Could you check a few things on this model? Use its own coordinates, in mm. Face numbers are marked on the shaded views. A direction names the side the tool comes from. Coordinates: 2 decimals unless noted, no trailing zeros. Write each loop counter-clockwise with the first axis right and the second up, starting at its lowest first coordinate (ties: lowest second). Pieces come first, ordered by that corner, then holes.
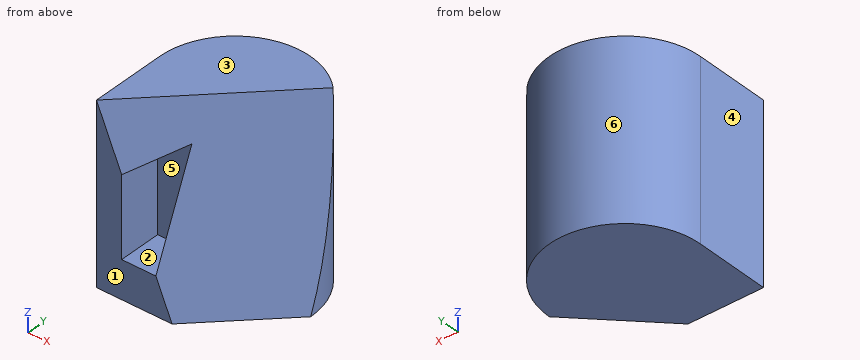
```python
from build123d import *

# Parameters (mm, degrees)
F1_DEPTH = 70
F6_DEPTH = 25


with BuildPart() as f1:
    # F0 (on Top) → F1 (new body)
    with BuildSketch(Plane.XY):
        with BuildLine():
            Line((-30, 0), (-30, -30))
            Line((-30, -30), (0, -30))
            Line((0, -30), (30, 0))
            ThreePointArc((30, 0), (0, 30), (-30, 0))
        make_face()
    extrude(amount=F1_DEPTH)

    # F4: sweep along a path in F3
    with BuildLine(Plane.XY.offset(70)) as f4_path:
        Line((-30, -30), (0, 0))
        Line((0, 0), (21.2132034356, 21.2132034356))
    # F2 (on face) → F4 (sweep, cut)
    with BuildSketch(Plane.XZ.offset(30)):
        Polygon((0, 70), (-30, 70), (0, 0), align=None)
    sweep(path=f4_path.line, mode=Mode.SUBTRACT)

    # F5 (on face) → F6 (cut)
    with BuildSketch(Plane.XZ.offset(30)):
        Polygon((-20, 46.6666666667), (-20, 15), (-6.4285714286, 15), (-6.4285714286, 55), align=None)
    extrude(amount=-F6_DEPTH, mode=Mode.SUBTRACT)

    # F7: sweep along a path in F7_path
    with BuildLine(Plane(origin=(-6.4285714286, -5, 55), x_dir=(0, 1, 0), z_dir=(-1, 0, 0))) as f7_path:
        Line((0, 0), (-7.8571428571, 0))
    # F6_face (on face) → F7 (sweep)
    with BuildSketch(Plane(origin=(-12.9512735327, -5, 32.9974160207), x_dir=(1, 0, 0), z_dir=(0, -1, 0))):
        Polygon((6.5227021041, 22.0025839793), (-7.0487264673, 13.669250646), (-7.0487264673, -17.9974160207), (6.5227021041, -17.9974160207), align=None)
    sweep(path=f7_path.line)


solid = f1.part
```
Item 1: If I drill on line 1 along X through (y, z) = (-17, 40); line 2 along Z through (x, y) = (-10, -18); line 3 along Y through (x, z) = (-10, 32), over which ranges is the centre line in solid material (lowest first)?
Item 2: I want a section at A-A, the plane z = 21. List the corners of the cut face in (x, y) for me.
Item 3: I want a section at B-B, the plane x = -14. List the corners of the cut face in (y, z) for me, then the cut area to 3 significant figures.
Item 4: Which directions (+Z, -Z, +X, -X, +Y, -Y) give clear straight access to the entire face, cutting with the end or side of a thin tool? Please do the marked faces 1 and 2.
Item 5: I want a section at C-C, the plane y = -16. List the corners of the cut face in (x, z) for me, then the cut area to 3 significant figures.
Item 6: If we mould it in two halves opening along X, with no side actions, what happens to the marked faces 3, 4, 5 and 6? For each: released by +X, released by -X, zero draft, split by the parting line, or undercut.
Item 7: Will these pins go through, and if not, where does the flat tip stop? pin 1 Ø5 at (x, z) = (5.5, 53.5) entering from -Y; pin 2 Ø10 at (x, z) = (-18, 46.5) entering from +Y; pin 3 Ø5 at (x, z) = (7.5, 41.5) entering from +Y.
Item 8: I want a section at D-D, the plane y = -6.5. List the corners of the cut face in (x, z) for me.
Taken from the geometry:
1. line 1: x = -30 to -20, -6.43 to -4.14
1. line 2: z = 0 to 15
1. line 3: y = -12.86 to 28.28
2. outline: (-30, -30) - (-20, -30) - (-20, -12.86) - (-6.43, -12.86) - (-6.43, -27.43) - (28.93, 7.93) arc R30 ccw to (-30, 0) - close
3. outline: (-30, 0) - (26.53, 0) - (26.53, 70) - (-14, 70) - (-22.42, 50.35) - (-12.86, 50.35) - (-12.86, 15) - (-30, 15) - close
3. area: 3,120 mm2
4. face 1: +Z, -Z, +X, -X, -Y
4. face 2: -Y
5. outline: (-30, 0) - (14, 0) - (-6.43, 47.67) - (-6.43, 15) - (-20, 15) - (-20, 46.67) - (-8.92, 53.47) - (-16, 70) - (-30, 70) - close
5. area: 1,550 mm2
6. face 3: zero draft
6. face 4: released by -X
6. face 5: undercut
6. face 6: split by the parting line
7. pin 1: stops at y = -4.29
7. pin 2: stops at y = 27.04
7. pin 3: stops at y = 29.58
8. outline: (-30, 0) - (23.5, 0) - (-6.5, 70) - (-30, 70) - close
